Check sheet for the modelled part. Datum: model origin and axes. Units: mm. Face numbers are marked on the shaded views. A direction names the side the tool comes from. Give positions to 0.01 mm unless a question says otherwise; leave off trailing zeros. Loops run counter-clockwise (first coordinate to the right, second up) from the corner with the lowest first, then second, coordinate; pieces in that order, holes last. Notation, with made-up numbers: (21.5, -3.5) -> (49.5, -3.5) arc R6 ccw to (49.5, 6.5) -> close; hole circle Ø3 at (65, -15.5). An arc over 180 degrees is marked (long way). Write each question's results on one line, items separated by ' | '. Start each with the question number.
Item 1: Scan lines: line 1 along X through (y, z) = (38, 0); line 2 along Z through (x, y) = (5.5, 73.5). Record each from-to range of solid material in increasing order.
Item 2: Access from +Z, -Z, +X, -X, +Y, -Y to the whole of each face (thin tool, end or side, straight path). Record for the marked faces 1 and 2.
Item 3: Gauge pin test, flat ends, axial feed: pin 1 Ø5 at (x, z) = (11, 50) entering from +Y; pin 2 Ø6.5 at (x, y) = (1, 73) entering from +Z; pin 3 Ø8 at (x, z) = (-0.5, 116.5) entering from +Y; pin 4 Ø5.5 at (x, z) = (0, 0) entering from +Y. Record the tip position at first contact, or that the pin passes through.
Item 4: Cross-section at B-B on z = 28. Enter the section's corners in (x, y).
Item 5: Cross-section at C-C on y = 32. Enter the section's corners in (x, z).
Item 6: Cross-section at A-A on y = 0. Enter the section's corners in (x, z).
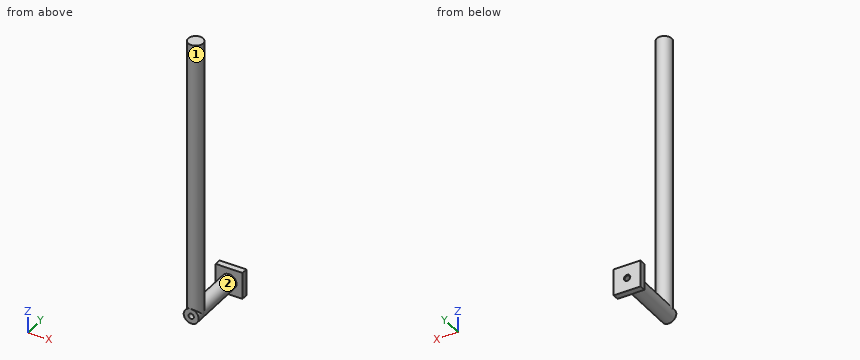
from build123d import *

# Parameters (mm, degrees)
SKETCH2_R                        = 9.5
BOSS_EXTRUDE1_DEPTH              = 355
SKETCH3_R                        = 9.5
BOSS_EXTRUDE2_DEPTH              = 70
BOSS_EXTRUDE3_START              = -9.5
SKETCH3_2_R                      = 9.5
BOSS_EXTRUDE3_DEPTH              = 9.5
SKETCH5_W                        = 34
SKETCH5_H                        = 34
BOSS_EXTRUDE4_DEPTH              = 8
M8X1_25_TAPPED_HOLE1_D           = 6.8
M8X1_25_TAPPED_HOLE1_CSINK_D     = 8.05
M8X1_25_TAPPED_HOLE1_CSINK_ANGLE = 90


with BuildPart() as part:
    # Sketch2 → Boss-Extrude1 (new body)
    with BuildSketch(Plane.XY):
        Circle(SKETCH2_R)
    extrude(amount=BOSS_EXTRUDE1_DEPTH)

    # Sketch3 → Boss-Extrude2 (add)
    with BuildSketch(Plane(origin=(0, 0, 0), x_dir=(1, 0, 0), z_dir=(0, 1, 0))):
        with Locations(Location((0, 0, 0), (0, 0, 180))):
            Circle(SKETCH3_R)
    extrude(amount=BOSS_EXTRUDE2_DEPTH)

    # Sketch3_2 → Boss-Extrude3 (add)
    with BuildSketch(Plane(origin=(0, 0, 0), x_dir=(1, 0, 0), z_dir=(0, 1, 0)).offset(BOSS_EXTRUDE3_START)):
        with Locations(Location((0, 0, 0), (0, 0, 270))):
            Circle(SKETCH3_2_R)
    extrude(amount=BOSS_EXTRUDE3_DEPTH)

    # Sketch5 → Boss-Extrude4 (add)
    with BuildSketch(Plane(origin=(0, 70, 0), x_dir=(1, 0, 0), z_dir=(0, 1, 0))):
        Rectangle(SKETCH5_W, SKETCH5_H)
    extrude(amount=BOSS_EXTRUDE4_DEPTH)

    # M8x1.25 Tapped Hole1 (through all)
    with Locations(Plane.ZX.offset(78)):
        with Locations((0, 0)):
            CounterSinkHole(M8X1_25_TAPPED_HOLE1_D / 2, M8X1_25_TAPPED_HOLE1_CSINK_D / 2, counter_sink_angle=M8X1_25_TAPPED_HOLE1_CSINK_ANGLE)


solid = part.part
Answer sheet:
1) line 1: x = -9.5 to -3.4, 3.4 to 9.5 | line 2: z = -17 to 17
2) face 1: +Z | face 2: none
3) pin 1: stops at y = 4.24 | pin 2: stops at z = 17 | pin 3: stops at y = 9.5 | pin 4: passes through
4) outline: circle Ø19 at (0, 0)
5) outline: circle Ø19 at (0, 0); hole circle Ø6.8 at (0, 0)
6) outline: (-9.5, 0) arc R9.5 ccw to (9.5, 0) -> (9.5, 355) -> (-9.5, 355) -> close; hole circle Ø6.8 at (0, 0)
